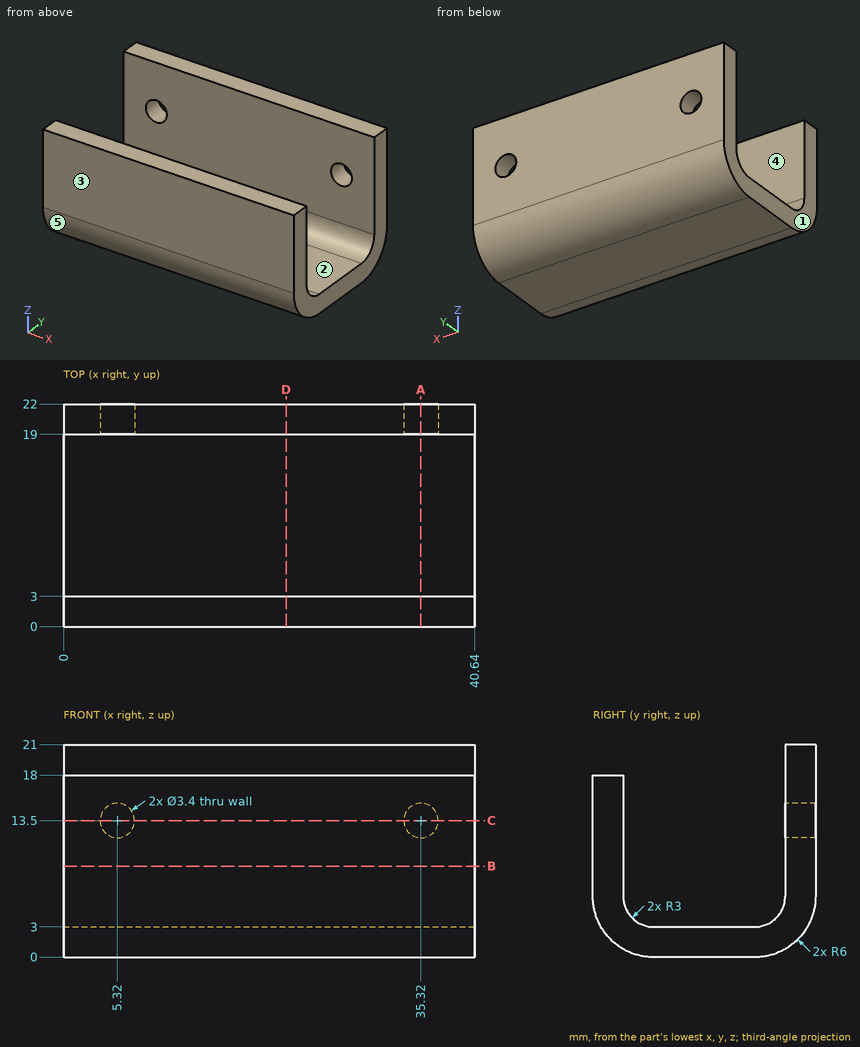
Geometry: see drawing. Coordinates: mm, zero at the bounding-box minimum. A direction names the side the tool comes from. Round coordinates to 2 decimals unless told otherwise and drop trailing zeros. Loops run counter-clockwise (first coordinate to the right, second up) from the corner with the lowest first, then second, coordinate; pieces in that order, holes last. Notation, with made-up numbers: M -37.5,22.25 L -0.5,22.25 A21 cw -0.5,53.25 Z; hole C 43,8.25 d6. An arc over 180 degrees is marked long. Use a Markdown table: item, result. Add a question column.
1. Pull-direction query (Y, two-part tool) for the marked faces 1, 2 and 3; classes: +Y half, -Y half, draft (parallel to the pull), parting line (faces both ways), or undercut.
2. Set-up query: the marked faces 4 and 5. Return all of +Z, -Z, +X, -X, +Y, -Y with unobstructed straight access to the full face (end or side cutting, diameter ignored); none if empty.
3. Cut plane B-B, the plane z = 9. Output: boundary loops of the cut face in (x, y).
4. Cut plane D-D, the plane x = 22. Output: boundary loops of the cut face in (y, z).
5. Contact query for flat-ended pins moving along their axis: pin 1 (3 mm diameter, centred on x = 14.5, y = 14, fed in from +Z); pin 2 (10 mm diameter, centred on x = 28, y = 13.5, fed in from +Z); pin 3 (3 mm diameter, centred on x = 5.32, z = 13.5, fed in from -Y); pin 4 (0.9 mm diameter, centred on x = 30, y = 1, fed in from +Z). Output: stop coordinate, or through.
6. Ray query, line 1 along X through (y, z) = (20, 13.5); line 2 along Y through (x, z) = (23.5, 17); line 3 along Z through (x, y) = (5.32, 21.4). Return the intervals inside material, ascending. Write a range as [from, to].
7. Cut plane A-A, the plane x = 35.32. Output: boundary loops of the cut face in (y, z).
8. Cut plane C-C, the plane z = 13.5. Output: boundary loops of the cut face in (x, y), and give its area (3 significant figures).
Solution:
| question | item | result |
|---|---|---|
| 1 | face 1 | draft |
| 1 | face 2 | undercut |
| 1 | face 3 | -Y half |
| 2 | face 4 | +Z, +X, -X |
| 2 | face 5 | -Z, +X, -X, -Y |
| 3 | outline | M 0,0 L 40.64,0 L 40.64,3 L 0,3 Z; M 0,19 L 40.64,19 L 40.64,22 L 0,22 Z |
| 4 | outline | M 0,6 A6 ccw 6,0 L 16,0 A6 ccw 22,6 L 22,21 L 19,21 L 19,6 A3 cw 16,3 L 6,3 A3 cw 3,6 L 3,18 L 0,18 Z |
| 5 | pin 1 | stops at z = 3 |
| 5 | pin 2 | stops at z = 4.34 |
| 5 | pin 3 | stops at y = 0 |
| 5 | pin 4 | stops at z = 18 |
| 6 | line 1 | x = [0, 3.62], [7.02, 33.62], [37.02, 40.64] |
| 6 | line 2 | y = [0, 3], [19, 22] |
| 6 | line 3 | z = [3.38, 11.8], [15.2, 21] |
| 7 | outline | M 0,6 A6 ccw 6,0 L 16,0 A6 ccw 22,6 L 22,11.8 L 19,11.8 L 19,6 A3 cw 16,3 L 6,3 A3 cw 3,6 L 3,18 L 0,18 Z; M 19,15.2 L 22,15.2 L 22,21 L 19,21 Z |
| 8 | outline | M 0,0 L 40.64,0 L 40.64,3 L 0,3 Z; M 0,19 L 3.62,19 L 3.62,22 L 0,22 Z; M 7.02,19 L 33.62,19 L 33.62,22 L 7.02,22 Z; M 37.02,19 L 40.64,19 L 40.64,22 L 37.02,22 Z |
| 8 | area | 223 mm2 |
